Here's the drawing with two shaded views (mm, measured from the low corner). I have some questions. Round coordinates to 2 decimals unless told otherwise and drop trailing zeros. Order: outer loops, then holes, each group sorted by start corner. A loop starts at its lowest first (then second) coordinate and runs counter-clockwise, first axis right, second up.
Q1. If I drill on line 1 (Y direction, x = 3.9, z = 0.35); line 2 (X direction, y = 6, z = 13.25); line 3 (X direction, y = 1.75, z = 4), over which ranges is the centre line in solid material (lowest first)?
Q2. We'd pull the mould along Y, two halves only. Please class the marked faces 1 and 2: pulls with the +Y half, pulls with the -Y half, needs draft (parallel to the pull), parting line crosses it, or undercut.
Q3. If we section it at C-C (z = 1.75): Please give me the cut outline in (x, y).
Q4. If we section it at A-A (x = 3.9): Please give me the cut outline in (y, z).
Q5. Will these pins go through, and if not, where does the flat tip stop? P1, Ø2, axis at x = 6.5, z = 13, coming from the +Y side; P2, Ø3, axis at x = 3.9, y = 3.9, coming from the -Z side; P3, Ø3, axis at x = 5, y = 4, coming from the -Z side.
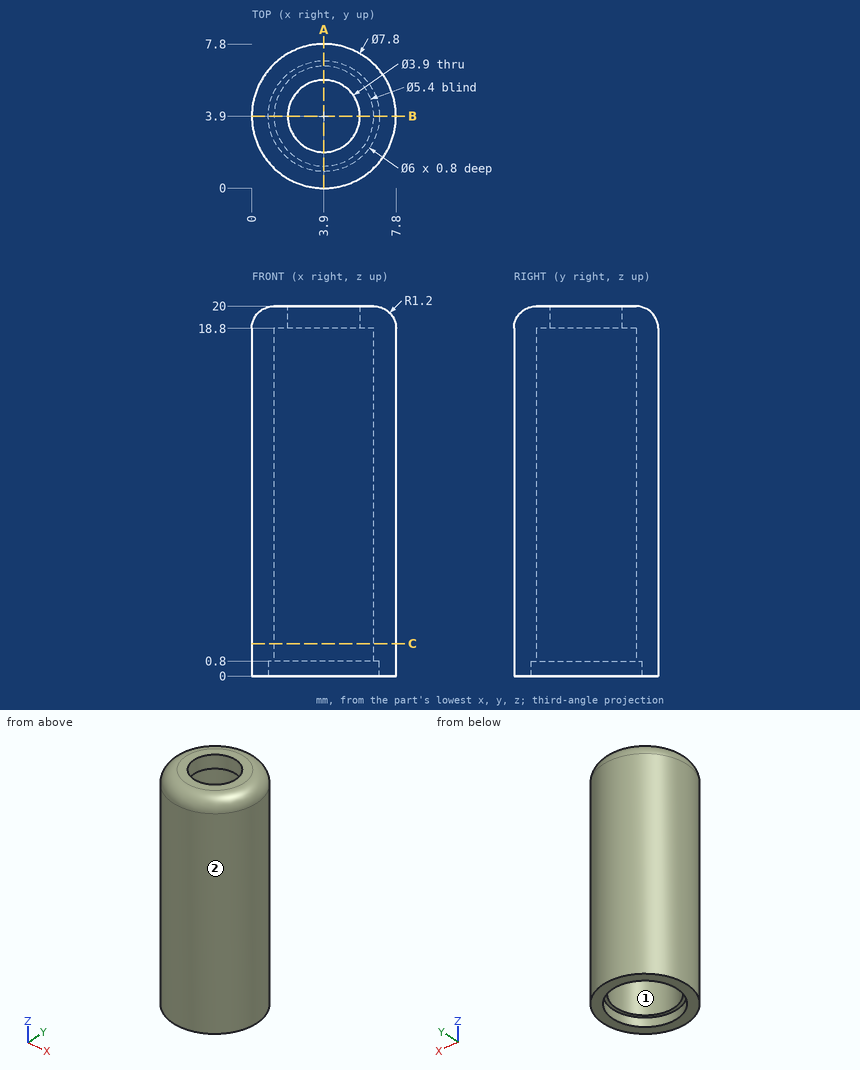
Solution:
1. line 1: y = 0 to 0.9, 6.9 to 7.8
1. line 2: x = 0.61 to 2.2, 5.6 to 7.19
1. line 3: x = 0.65 to 2.27, 5.53 to 7.15
2. face 1: undercut
2. face 2: parting line crosses it
3. outline: circle Ø7.8 at (3.9, 3.9); hole circle Ø5.4 at (3.9, 3.9)
4. outline: (0, 0) - (0.9, 0) - (0.9, 0.8) - (1.2, 0.8) - (1.2, 18.8) - (1.95, 18.8) - (1.95, 20) - (1.2, 20) arc R1.2 ccw to (0, 18.8) - close; (5.85, 18.8) - (6.6, 18.8) - (6.6, 0.8) - (6.9, 0.8) - (6.9, 0) - (7.8, 0) - (7.8, 18.8) arc R1.2 ccw to (6.6, 20) - (5.85, 20) - close
5. P1: stops at y = 7.46
5. P2: passes through
5. P3: stops at z = 18.8
